Geometry: final body of the model. Coordinates: model frame, mm. A direction names the side the tool comes from. Give positions to 0.01 mm unless a question says otherwise; leave off trailing zeros. Order: outer loops, then holes, each group sorted by start corner. A loop starts at its lowest first (then second) coordinate and runs counter-clockwise, first axis right, second up. Notation, with made-up numbers: M 81.5,50 L 105.5,50 A21 cw 105.5,63 Z; hole C 18.25,-22 d6. An arc over 180 degrees is marked long. Write item = value, one per line. Start each with the question number.
from build123d import *

# Parameters (mm, degrees)
F0_W           = 29
F0_H           = 6
F1_DEPTH       = 8
F2_R           = 5
F3_DEPTH       = 6
F5_D           = 3.2
F5_DEPTH       = 10
F5_CSINK_D     = 5.5
F5_CSINK_ANGLE = 90
F5_TIP         = 0.9613769904
F6_T1_DEPTH    = 18.2867319519


# Not quite as in the source:
# - a fillet or chamfer that OpenCascade refuses, or shapes differently, is made with other operations: its cross-section is extruded or revolved along the edge and cut away or added


with BuildPart() as f1:
    # F0 (on Front) → F1 (new body)
    with BuildSketch(Plane.XZ):
        with Locations((14.5, 3)):
            Rectangle(F0_W, F0_H)
    extrude(amount=F1_DEPTH)

    # F2 (on face) → F3 (cut)
    with BuildSketch(Plane(origin=(0, 0, 0), x_dir=(-1, 0, 0), z_dir=(0, 1, 0))):
        with Locations((-14.5, 0)):
            Circle(F2_R)
    extrude(amount=-F3_DEPTH, mode=Mode.SUBTRACT)

    # F5
    with Locations(Plane.XY.offset(6)):
        with Locations((4.75, -4), (24.25, -4)):
            CounterSinkHole(F5_D / 2, F5_CSINK_D / 2, depth=F5_DEPTH, counter_sink_angle=F5_CSINK_ANGLE)
            with Locations((0, 0, -(F5_DEPTH + F5_TIP / 2))):  # 118° drill point
                Cone(0, F5_D / 2, F5_TIP, mode=Mode.SUBTRACT)

    # F6: chamfer of 2 on 2 edges, made by hand

    # F6_s2 → F6_t1 (cut)
    with BuildSketch(Plane.XZ.offset(-5.1433659759)):
        Polygon((27, 6), (29, 4), (29, 6), align=None)
        Polygon((0, 4), (2, 6), (0, 6), align=None)
    extrude(amount=F6_T1_DEPTH, mode=Mode.SUBTRACT)


solid = f1.part
1) Cut plane A-A (x = 4.75). Return loops of the section in (y, z).
2) Cut plane C-C (x = 14.5). Return loops of the section in (y, z).
3) Cut plane B-B (z = 3.05). Return loops of the section in (x, y).
4) Cut plane D-D (y = -3.25). Give the number of separate pieces and of enclosed holes in the cut face, plus the area to 3 significant figures.
5) Access query for faces 5 (the cylindrical face through (14.4, -3, 5)), 6 (the flat face through (0, -4, 2)). Directions: +Z, -Z, +X, -X, +Y, -Y. A direction counts if a zero-diameter tool reaches every point of the face in a straight line with its end or side. Return the directions, or none.
6) Ray query, L1, parallel to Y at x = 4.75, z = 1.75; L2, parallel to X at y = -4, z = 2.65; L3, parallel to X at y = -4, z = 2.3. Return the intervals inside material, ascending.
7) Draft query along X for faces 1 (the flat face through (29, -4, 2)), 2 (the cylindrical face through (6, -3, 2)), 3 (the flat face through (14, -4, 6)), 4 (the flat face through (15, -6, 2)). Return one class per face: pulls with the +X half, pulls with the -X half, needs draft (parallel to the pull), parting line crosses it, or undercut.
8) Pin query (flat end, axial travel): pin 1 Ø2.5 at (x, z) = (17, 2.5) entering from +Y; pin 2 Ø1 at (y, z) = (-3, 1) entering from -X. Return the tip coordinate at first contact, or that it passes through.
Reply:
q1.outline = M -8,0 L -5.6,0 L -5.6,4.85 L -6.75,6 L -8,6 Z; M -2.4,0 L 0,0 L 0,6 L -1.25,6 L -2.4,4.85 Z
q2.outline = M -8,0 L -6,0 L -6,5 L 0,5 L 0,6 L -8,6 Z
q3.outline = M 0,-8 L 29,-8 L 29,0 L 18.46,0 L 18.46,-6 L 10.54,-6 L 10.54,0 L 0,0 Z; hole C 4.75,-4 d3.2; hole C 24.25,-4 d3.2
q4.separate_pieces = 3
q4.enclosed_holes = 0
q4.area = 93.9 mm²
q5.face_5 = -Z, +Y
q5.face_6 = +Z, -Z, -X, +Y, -Y
q6.L1 = -8 to -5.6, -2.4 to 0
q6.L2 = 0 to 3.15, 6.35 to 10.26, 18.74 to 22.65, 25.85 to 29
q6.L3 = 0 to 3.15, 6.35 to 10.06, 18.94 to 22.65, 25.85 to 29
q7.face_1 = pulls with the +X half
q7.face_2 = undercut
q7.face_3 = needs draft
q7.face_4 = undercut
q8.pin_1 = -6
q8.pin_2 = 0
